Work out the finished part from the listing and answer in its coordinate system (mm). Face numbers are marked on the shaded views. A direction names the side the tool comes from. Give positions to 0.01 mm unless a question says otherwise; leave off trailing zeros. Write each loop counter-clockwise with the first axis right and the second up, starting at its lowest first coordinate (ties: lowest second). Pieces come first, ordered by that corner, then holes. Notation, with made-up numbers: (63.5, -23) - (113.5, -23) arc R14 ccw to (113.5, 0) - close; hole circle Ø2 at (89, 78.25). An arc over 180 degrees is marked (long way). Write each question's results on one line, items separated by ' | '. Start each with the question number.
from build123d import *

# Parameters (mm, degrees)
SKETCH_2_W          = 30
SKETCH_2_H          = 30
CUT_EXTRUDE_1_DEPTH = 7.5


with BuildPart() as part:
    # Sketch 1 → Revolve 1 (revolve)
    with BuildSketch(Plane.XY, mode=Mode.PRIVATE) as revolve_1_sk:
        Polygon((-7.5, 0), (-7.5, 5), (-5.5, 5), (-5.5, 6.5), (-4.922649731, 7.5), (0, 7.5), (0, 4), (24.233, 4), (25, 3.233), (25, 0), align=None)
    revolve(revolve_1_sk.sketch.rotate(Axis((25, 0, 0), (-1, 0, 0)), 270), axis=Axis((25, 0, 0), (-1, 0, 0)))

    # Sketch 2 → Cut-Extrude 1 (cut)
    with BuildSketch(Plane(origin=(0, 0, 0), x_dir=(0, 0, -1), z_dir=(1, 0, 0))):
        Rectangle(SKETCH_2_W, SKETCH_2_H)
        Polygon((-6.5, 3.75277675), (-6.5, -3.75277675), (0, -7.5), (6.5, -3.75277675), (6.5, 3.75277675), (0, 7.5), align=None, mode=Mode.SUBTRACT)
    extrude(amount=-CUT_EXTRUDE_1_DEPTH, mode=Mode.SUBTRACT)


solid = part.part
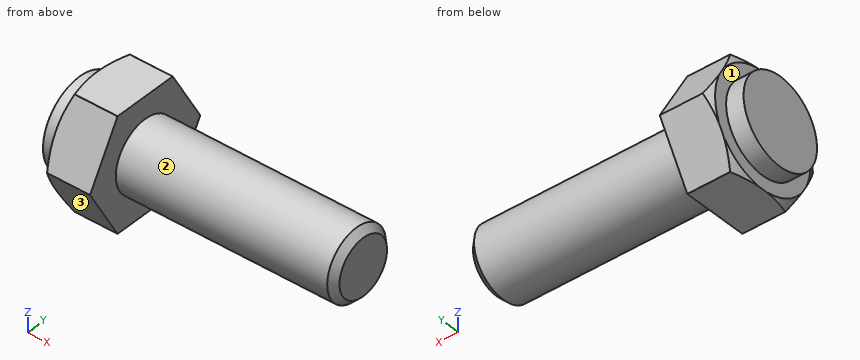
Q1. A tool of negligible diameter and unlimited length cuts with its end or side. For the marked faces 1, 2 and 3, from which of +Z, -Z, +X, -X, +Y, -Y can it reach the whole face along a straight path? Write none if from no direction.
Q2. Given pin 1 (2 mm diameter, centred on x = 16.5, y = -4, fed in from +Z); pin 2 (2 mm diameter, centred on y = 5.5, z = -4, fed in from -X); pin 3 (2 mm diameter, centred on y = 0.5, z = -4.5, fed in from +X), each flat-ended and moving along its own axis, determine where each tip first touches the part or whether it passes through.
Q3. Consider L1, parallel to Y at x = 7, z = 0; L2, parallel to X at y = -4.5, z = -0.25; L3, parallel to X at y = 6, z = -0.75. Determine where each line is inside the solid, lowest interval first.
Q4. A cutting plane is placed at A-A, the plane x = 18.5. Write down the section's boundary in (y, z).
Result:
1) face 1: -X | face 2: +X | face 3: -Z, +X, -X, -Y
2) pin 1: stops at z = 2.65 | pin 2: stops at x = -5.5 | pin 3: stops at x = 24.71
3) L1: y = -4 to 4 | L2: x = -7.5 to 0 | L3: x = -5.5 to 0
4) outline: circle Ø8 at (0, 0)
